Work out the finished part from the listing and answer in its coordinate system (mm). Face numbers are marked on the shaded views. Round coordinates to 2 decimals unless told otherwise and drop trailing zeros. Loops run counter-clockwise (first coordinate to the right, second up) from the corner with the lowest first, then second, coordinate; pieces in that order, holes last.
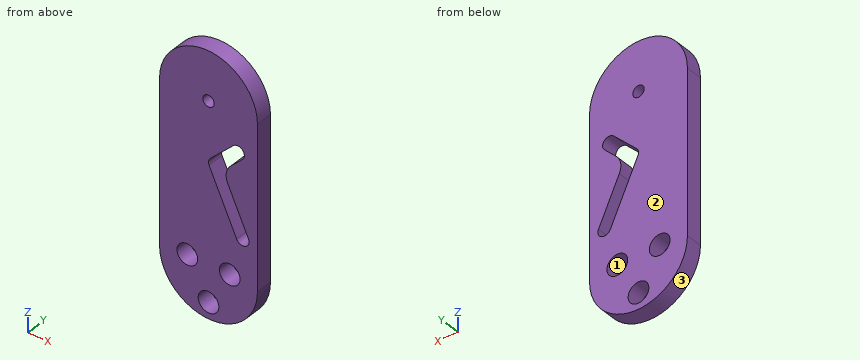
from build123d import *

# Parameters (mm, degrees)
SKETCH1_R           = 3.175
SKETCH1_R_2         = 1.75
BOSS_EXTRUDE1_DEPTH = 5
FILLET1_R           = 5


with BuildPart() as part:
    # Sketch1 → Boss-Extrude1 (new body)
    with BuildSketch(Plane(origin=(0, 0, 0), x_dir=(1, 0, 0), z_dir=(0, 1, 0))):
        with BuildLine():
            Line((15, 0), (15, 50))
            ThreePointArc((15, 50), (0, 65), (-15, 50))
            Line((-15, 50), (-15, 0))
            ThreePointArc((-15, 0), (0, -15), (15, 0))
        make_face()
        with Locations((6.5, 48.741669751)):
            Circle(SKETCH1_R, mode=Mode.SUBTRACT)
        with Locations((-6.5, 48.741669751)):
            Circle(SKETCH1_R, mode=Mode.SUBTRACT)
        with Locations((0, 60)):
            Circle(SKETCH1_R, mode=Mode.SUBTRACT)
        Circle(SKETCH1_R_2, mode=Mode.SUBTRACT)
        with BuildLine():
            ThreePointArc((7.585786438, 9.807118725), (10.414213562, 9.807118725), (10.414213562, 12.63554585))
            Line((10.414213562, 12.63554585), (4.397206201, 18.652553211))
            Line((4.397206201, 18.652553211), (12.25773045, 35.509501863))
            ThreePointArc((12.25773045, 35.509501863), (11.2903514, 38.167353961), (8.632499302, 37.19997491))
            Line((8.632499302, 37.19997491), (0.180134067, 19.07381917))
            ThreePointArc((0.180134067, 19.07381917), (0.023134135, 17.881286291), (0.578536079, 16.814369084))
            Line((0.578536079, 16.814369084), (7.585786438, 9.807118725))
        make_face(mode=Mode.SUBTRACT)
    extrude(amount=BOSS_EXTRUDE1_DEPTH)

    # Fillet1
    fillet1_edges = [part.edges().sort_by_distance(p)[0] for p in [
        (4.397206201, 2.5, -18.652553211),
    ]]
    fillet(fillet1_edges, radius=FILLET1_R)


solid = part.part
Item 1: Section C-C, the plane y = 3.2 is taken. State how many separate pieces and enclosed holes the cut face has, plus the area to 3 significant figures.
Item 2: Section D-D, the plane z = 9 is taken. Give the vertices of the cut face in (x, y), plus the area to 3 significant figures.
Item 3: Each of these flat-tipped pins is pushed along its axis until it touches: P1, Ø1.5, axis at x = -2.5, y = 2, coming from the +Z side; P2, Ø8, axis at x = -8.5, z = -4, coming from the -Y side; P3, Ø4, axis at x = 0, z = -60, coming from the +Y side. Where does it stop, or does it pass through?
Item 4: Determine the mould class of the marked faces 1, 2 and 3 for opening direction X: pulls with the +X half, pulls with the -X half, needs draft (parallel to the pull), parting line crosses it, or undercut.
Item 5: Straight lines are drawn through the part: line 1 (Z direction, x = 8.5, y = 4.5); line 2 (Z direction, x = 6.5, y = 1.8); line 3 (Z direction, x = 2, y = 4.25). For each, find the intervals that lie inside material, in ascending order.
Item 6: Section A-A, the plane x = -6.5 is taken. Give the vertices of the cut face in (y, z).
Item 7: Section B-B, the plane z = -34 is taken. Give the vertices of the cut face in (x, y).
Answer below:
1. separate pieces: 1
1. enclosed holes: 5
1. area: 1,970 mm2
2. outline: (-12, 0) - (12, 0) - (12, 5) - (-12, 5) - close
2. area: 120 mm2
3. P1: stops at z = 14.9
3. P2: stops at y = 0
3. P3: passes through
4. face 1: undercut
4. face 2: needs draft
4. face 3: parting line crosses it
5. line 1: z = -62.36 to -51.21, -46.28 to -36.92, -27.45 to -14.55, -9.28 to 12.36
5. line 2: z = -63.52 to -51.92, -45.57 to -32.63, -23.16 to -16.59, -10.89 to 13.52
5. line 3: z = -64.87 to -62.47, -57.53 to -22.98, -15.39 to 14.87
6. outline: (0, -63.52) - (5, -63.52) - (5, -51.92) - (0, -51.92) - close; (0, -45.57) - (5, -45.57) - (5, 13.52) - (0, 13.52) - close
7. outline: (-15, 0) - (7.14, 0) - (7.14, 5) - (-15, 5) - close; (11.55, 0) - (15, 0) - (15, 5) - (11.55, 5) - close
